```python
from build123d import *

# Parameters (mm, degrees)
SKETCH1_R           = 3.175
BOSS_EXTRUDE1_DEPTH = 6.35


with BuildPart() as part:
    # Sketch1 → Boss-Extrude1 (new body)
    with BuildSketch(Plane(origin=(0, 0, 0), x_dir=(1, 0, 0), z_dir=(0, 1, 0))):
        with BuildLine():
            Line((-49.784, 44.45), (49.784, 44.45))
            Line((49.784, 44.45), (49.784, 38.1))
            Line((49.784, 38.1), (43.434, 38.1))
            Line((43.434, 38.1), (43.434, 25.4))
            Line((43.434, 25.4), (49.784, 25.4))
            Line((49.784, 25.4), (49.784, 6.35))
            Line((49.784, 6.35), (43.434, 6.35))
            Line((43.434, 6.35), (43.434, -6.35))
            Line((43.434, -6.35), (49.784, -6.35))
            Line((49.784, -6.35), (49.784, -25.4))
            Line((49.784, -25.4), (43.434, -25.4))
            Line((43.434, -25.4), (43.434, -38.1))
            Line((43.434, -38.1), (49.784, -38.1))
            Line((49.784, -38.1), (49.784, -44.45))
            ThreePointArc((49.784, -44.45), (0, -94.234), (-49.784, -44.45))
            Line((-49.784, -44.45), (-49.784, -38.1))
            Line((-49.784, -38.1), (-43.434, -38.1))
            Line((-43.434, -38.1), (-43.434, -25.4))
            Line((-43.434, -25.4), (-49.784, -25.4))
            Line((-49.784, -25.4), (-49.784, -6.35))
            Line((-49.784, -6.35), (-43.434, -6.35))
            Line((-43.434, -6.35), (-43.434, 6.35))
            Line((-43.434, 6.35), (-49.784, 6.35))
            Line((-49.784, 6.35), (-49.784, 25.4))
            Line((-49.784, 25.4), (-43.434, 25.4))
            Line((-43.434, 25.4), (-43.434, 38.1))
            Line((-43.434, 38.1), (-49.784, 38.1))
            Line((-49.784, 38.1), (-49.784, 44.45))
        make_face()
        with Locations((0, -69.342)):
            Circle(SKETCH1_R, mode=Mode.SUBTRACT)
    extrude(amount=BOSS_EXTRUDE1_DEPTH)


solid = part.part
```
CAD build for the part. Positions are in the model's coordinates, mm. A direction names the side the tool comes from. Round coordinates to 2 decimals unless told otherwise and drop trailing zeros. Order: outer loops, then holes, each group sorted by start corner. A loop starts at its lowest first (then second) coordinate and runs counter-clockwise, first axis right, second up. Notation, with made-up numbers: (-7.5, -28.75) - (47.5, -28.75) arc R37 cw to (47.5, 7.25) - close; hole circle Ø9 at (42.5, 79). An arc over 180 degrees is marked (long way). Answer in a Markdown table with one row per item. Add a question column.
(1) Probe L1, parallel to Z at x = 0, y = 4.5; L2, parallel to X at y = 2.25, z = 4; L3, parallel to Z at x = 11.5, y = 0.75. List the from-to ranges inside material, lowest first. Write a range as [from, to].
(2) Drop flat-ended pins along their axis: pin 1 Ø3 at (y, z) = (4, 1.5) entering from +X; pin 2 Ø12 at (x, z) = (13, -21) entering from -Y; pin 3 Ø1.9 at (x, y) = (-46, 3.5) entering from +Z; pin 4 Ø3 at (x, y) = (46, 4.5) entering from +Z. Give the stop position or say it passes through.
(3) Band-saw the part on A-A on x = 0. List the corners of the cut face in (y, z), and give its area (3 significant figures).
(4) Band-saw the part on D-D on x = 30. List the corners of the cut face in (y, z).
(5) Band-saw the part on C-C on z = -31.5. List the corners of the cut face in (x, y), and give its area (3 significant figures).
(6) 3-axis set-ups, long thin cutter, end or side, ignore diameter. For faces 1 (the face through (-49.784, 3, -16)), 2 (the face through (43.434, 3, 0)), 3 (the face through (-47, 3, 38.1)): which of +Z, -Z, +X, -X, +Y, -Y reach the whole face in a straight line?
(7) Mould opens along Z. For faces 4 (the face through (47, 3, -25.4)), 5 (the face through (-49.784, 3, 41)) say: +Z half, -Z half, draft (parallel to the pull), parting line (faces both ways), or undercut.
Data:
| question | item | result |
|---|---|---|
| 1 | L1 | z = [-44.45, 66.17], [72.52, 94.23] |
| 1 | L2 | x = [-43.43, 43.43] |
| 1 | L3 | z = [-44.45, 92.89] |
| 2 | pin 1 | stops at x = 43.43 |
| 2 | pin 2 | stops at y = 0 |
| 2 | pin 3 | stops at z = 65.64 |
| 2 | pin 4 | stops at z = 66.77 |
| 3 | outline | (0, -44.45) - (6.35, -44.45) - (6.35, 66.17) - (0, 66.17) - close; (0, 72.52) - (6.35, 72.52) - (6.35, 94.23) - (0, 94.23) - close |
| 3 | area | 840 mm^2 |
| 4 | outline | (0, -44.45) - (6.35, -44.45) - (6.35, 84.18) - (0, 84.18) - close |
| 5 | outline | (-43.43, 0) - (43.43, 0) - (43.43, 6.35) - (-43.43, 6.35) - close |
| 5 | area | 552 mm^2 |
| 6 | face 1 | +Z, -Z, -X, +Y, -Y |
| 6 | face 2 | +X, +Y, -Y |
| 6 | face 3 | -X, +Y, -Y |
| 7 | face 4 | undercut |
| 7 | face 5 | draft |
